from build123d import *

# Parameters (mm, degrees)
RESSALTO_EXTRUS_O1_DEPTH = 3


with BuildPart() as part:
    # Esboço1 → Ressalto-extrusão1 (new body)
    with BuildSketch(Plane.XY):
        with BuildLine():
            Line((-38.5, -4.5), (-7.5, -4.5))
            ThreePointArc((-7.5, -4.5), (-5.378679656, -3.621320344), (-4.5, -1.5))
            Line((-4.5, -1.5), (-4.5, 0))
            ThreePointArc((-4.5, 0), (-3.181980515, 3.181980515), (0, 4.5))
            Line((0, 4.5), (1.5, 4.5))
            ThreePointArc((1.5, 4.5), (3.621320344, 5.378679656), (4.5, 7.5))
            Line((4.5, 7.5), (4.5, 38.5))
            ThreePointArc((4.5, 38.5), (3.621320344, 40.621320344), (1.5, 41.5))
            Line((1.5, 41.5), (0, 41.5))
            ThreePointArc((0, 41.5), (-3.181980515, 42.818019485), (-4.5, 46))
            Line((-4.5, 46), (-4.5, 47.5))
            ThreePointArc((-4.5, 47.5), (-5.378679656, 49.621320344), (-7.5, 50.5))
            Line((-7.5, 50.5), (-38.5, 50.5))
            ThreePointArc((-38.5, 50.5), (-40.621320344, 49.621320344), (-41.5, 47.5))
            Line((-41.5, 47.5), (-41.5, 46))
            ThreePointArc((-41.5, 46), (-42.818019485, 42.818019485), (-46, 41.5))
            Line((-46, 41.5), (-52.5, 41.5))
            ThreePointArc((-52.5, 41.5), (-54.621320344, 40.621320344), (-55.5, 38.5))
            ThreePointArc((-55.5, 38.5), (-58, 36), (-60.5, 38.5))
            ThreePointArc((-60.5, 38.5), (-58.156854249, 44.156854249), (-52.5, 46.5))
            Line((-52.5, 46.5), (-46.5, 46.5))
            Line((-46.5, 46.5), (-46.5, 47.5))
            ThreePointArc((-46.5, 47.5), (-44.156854249, 53.156854249), (-38.5, 55.5))
            Line((-38.5, 55.5), (-7.5, 55.5))
            ThreePointArc((-7.5, 55.5), (-1.843145751, 53.156854249), (0.5, 47.5))
            Line((0.5, 47.5), (0.5, 46.5))
            Line((0.5, 46.5), (1.5, 46.5))
            ThreePointArc((1.5, 46.5), (7.156854249, 44.156854249), (9.5, 38.5))
            Line((9.5, 38.5), (9.5, 7.5))
            ThreePointArc((9.5, 7.5), (7.156854249, 1.843145751), (1.5, -0.5))
            Line((1.5, -0.5), (0.5, -0.5))
            Line((0.5, -0.5), (0.5, -1.5))
            ThreePointArc((0.5, -1.5), (-1.843145751, -7.156854249), (-7.5, -9.5))
            Line((-7.5, -9.5), (-38.5, -9.5))
            ThreePointArc((-38.5, -9.5), (-44.156854249, -7.156854249), (-46.5, -1.5))
            Line((-46.5, -1.5), (-46.5, -0.5))
            Line((-46.5, -0.5), (-52.5, -0.5))
            ThreePointArc((-52.5, -0.5), (-58.156854249, 1.843145751), (-60.5, 7.5))
            ThreePointArc((-60.5, 7.5), (-58, 10), (-55.5, 7.5))
            ThreePointArc((-55.5, 7.5), (-54.621320344, 5.378679656), (-52.5, 4.5))
            Line((-52.5, 4.5), (-46, 4.5))
            ThreePointArc((-46, 4.5), (-42.818019485, 3.181980515), (-41.5, 0))
            Line((-41.5, 0), (-41.5, -1.5))
            ThreePointArc((-41.5, -1.5), (-40.621320344, -3.621320344), (-38.5, -4.5))
        make_face()
    extrude(amount=RESSALTO_EXTRUS_O1_DEPTH)


solid = part.part
Part model, mm, in its own coordinate system. A direction names the side the tool comes from. Give positions to 0.01 mm unless a question says otherwise; leave off trailing zeros. Write each loop counter-clockwise with the first axis right and the second up, starting at its lowest first coordinate (ties: lowest second). Pieces come first, ordered by that corner, then holes.
1) Pin check, flat tips, straight feed: pin 1 (0.8 mm diameter, centred on x = 1, z = 1, fed in from -Y); pin 2 (1.5 mm diameter, centred on x = -41, z = 1.5, fed in from +Y); pin 3 (1.2 mm diameter, centred on x = 0.5, z = 2, fed in from +Y). Stop position of each tip, or through.
Resolved:
pin 1: stops at y = -0.5
pin 2: stops at y = 55.31
pin 3: stops at y = 50.54
2) Which spindle directions (+Z, -Z, +X, -X, +Y, -Y) get a long thin tool onto all of the face, cutting with end or side? Do faces 1 (the face through (-4.5, -1, 1)), 2 (the face through (-1.781, -7.094, 1.479)). Say none if no direction does.
Resolved:
face 1: +Z, -Z
face 2: +Z, -Z, +X, -Y
3) Cut at C-C on y = 27.5. Write the cut outline in (x, z), then the cut area to 3 significant figures.
Resolved:
outline: (4.5, 0) - (9.5, 0) - (9.5, 3) - (4.5, 3) - close
area: 15.0 mm2
4) Cut at A-A on x = -28. Write the cut outline in (y, z), then the cut area to 3 significant figures.
Resolved:
outline: (-9.5, 0) - (-4.5, 0) - (-4.5, 3) - (-9.5, 3) - close; (50.5, 0) - (55.5, 0) - (55.5, 3) - (50.5, 3) - close
area: 30.0 mm2
5) Two-plate mould, pull along Y, no slides. Class faces 3 (the face through (-44.219, 53.094, 1.479)), 4 (the face through (-42.783, 42.853, 1.479)), 5 (the face through (7.219, 1.906, 1.479)): released by +Y, released by -Y, zero draft, split by the parting line, or undercut.
Resolved:
face 3: released by +Y
face 4: undercut
face 5: released by -Y
6) Cut at B-B on x = -6. Write the cut outline in (y, z).
Resolved:
outline: (-9.36, 0) - (-4.1, 0) - (-4.1, 3) - (-9.36, 3) - close; (50.1, 0) - (55.36, 0) - (55.36, 3) - (50.1, 3) - close
7) Probe L1, parallel to X at y = 47.5, z = 2.1; L2, parallel to Y at x = -13, z = 1; L3, parallel to Y at x = -41, z = 0.8. List the from-to ranges inside material, lowest first.
Resolved:
L1: x = -46.5 to -41.5, -4.5 to 0.5
L2: y = -9.5 to -4.5, 50.5 to 55.5
L3: y = -9.1 to -3.16, 49.16 to 55.1
